Here's how the part is built. I have some questions about the finished solid (model axes, mm). Face numbers are marked on the shaded views. A direction names the side the tool comes from. Give positions to 0.01 mm unless a question says otherwise; leave off trailing zeros. Order: outer loops, then holes, each group sorted by start corner. A loop starts at its lowest first (then second) coordinate and runs counter-clockwise, first axis right, second up.
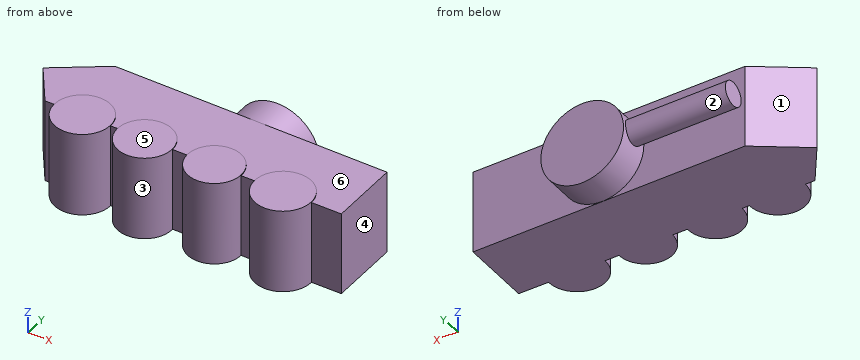
from build123d import *

# Parameters (mm, degrees)
F1_DEPTH = 39.081264
F2_R     = 13.086834
F2_R_2   = 12.762308
F2_R_3   = 12.541297
F2_R_4   = 13.219685
F3_DEPTH = 39.425768
F4_R     = 19.429487
F5_DEPTH = 14.579227
F6_R     = 5.692601
F7_DEPTH = 52.206531


with BuildPart() as f1:
    # F0 (on Top) → F1 (new body)
    with BuildSketch(Plane.XY):
        Polygon((-52.925434, 16.347141), (-76.083884, 0), (-63.54259, -17.766833), (74.829757, -16.512707), (74.829757, 16.347141), align=None)
    extrude(amount=F1_DEPTH)

    # F2 (on Top) → F3 (join)
    with BuildSketch(Plane.XY):
        with Locations((-45.984775, -17.766833)):
            Circle(F2_R)
        with Locations((-16.72174, -17.766833)):
            Circle(F2_R_2)
        with Locations((15.467599, -16.930744)):
            Circle(F2_R_3)
        with Locations((47.656953, -16.930744)):
            Circle(F2_R_4)
    extrude(amount=F3_DEPTH)

    # F4 (on face) → F5 (join)
    with BuildSketch(Plane(origin=(0, 16.347141, 0), x_dir=(-1, 0, 0), z_dir=(0, 1, 0))):
        with Locations((-14.022259, 19.540632)):
            Circle(F4_R)
    extrude(amount=F5_DEPTH)

    # F6 (on Right) → F7 (join)
    with BuildSketch(Plane.YZ):
        with Locations((23.680674, 21.317706)):
            Circle(F6_R)
    extrude(amount=-F7_DEPTH)


solid = f1.part
Q1. I'm going to push flat-ended pins straight in: P1, Ø10, axis at y = -8, z = 21.5, coming from the -X side; P2, Ø1.5, axis at y = 15.5, z = 16.5, coming from the -X side; P3, Ø8, axis at x = 5.5, z = 7.5, coming from the -Y side; P4, Ø10, axis at x = 5, y = -5, coming from the +Z side. Where does each tip first touch, or does it pass through?
Filled sheet:
P1: stops at x = -73.97
P2: stops at x = -55.19
P3: stops at y = -27.96
P4: stops at z = 39.43
Q2. For the marked faces 5 and 6, which set-ups out of +Z, -Z, +X, -X, +Y, -Y let a thin tool reach every point of the face, with its end or its side?
Filled sheet:
face 5: +Z, +X, -X, +Y, -Y
face 6: +Z, +Y
Q3. If we section it at B-B on x = -45: List the corners of the cut face in (y, z) for me, plus the area to 3 significant figures.
Filled sheet:
outline: (-30.82, 0) - (16.35, 0) - (16.35, 39.08) - (-4.72, 39.08) - (-4.72, 39.43) - (-30.82, 39.43) - close; circle Ø11.39 at (23.68, 21.32)
area: 1,950 mm2
Q4. If we section it at C-C on z = 32: List the corners of the cut face in (x, y) for me, plus the area to 3 significant figures.
Filled sheet:
outline: (-76.08, 0) - (-63.54, -17.77) - (-59.07, -17.73) arc R13.09 ccw (long way) to (-32.9, -17.49) - (-29.48, -17.46) arc R12.76 ccw (long way) to (-3.97, -17.23) - (2.93, -17.16) arc R12.54 ccw to (28.01, -16.94) - (34.44, -16.88) arc R13.22 ccw (long way) to (60.87, -16.64) - (74.83, -16.51) - (74.83, 16.35) - (28.93, 16.35) - (28.93, 30.93) - (-0.89, 30.93) - (-0.89, 16.35) - (-52.93, 16.35) - close
area: 6,260 mm2
Q5. Thinking about a two-plate mould opening in X: for the marked faces 1, 2, 3 and 4, which applies, released by +X, released by -X, zero draft, split by the parting line, or undercut?
Filled sheet:
face 1: released by -X
face 2: zero draft
face 3: undercut
face 4: released by +X
Q6. If we section it at D-D on x = -17: List the corners of the cut face in (y, z) for me, plus the area to 3 significant figures.
Filled sheet:
outline: (-30.53, 0) - (16.35, 0) - (16.35, 39.08) - (-5.01, 39.08) - (-5.01, 39.43) - (-30.53, 39.43) - close; circle Ø11.39 at (23.68, 21.32)
area: 1,940 mm2
Q7. I need wall thicknesses on L1, parallel to X at y = -24, z = 27.5; L2, parallel to Y at x = -15.5, z = 17.5; L3, parallel to X at y = -25, z = 35. Which ranges of each line are inside material? Lowest first, please.
Filled sheet:
L1: x = -57.49 to -34.48, -27.86 to -5.59, 5.11 to 25.83, 36.49 to 58.83
L2: y = -30.47 to 16.35, 19.46 to 27.9
L3: x = -56.89 to -35.08, -27.24 to -6.21, 5.87 to 25.07, 37.19 to 58.13
Q8. If we section it at A-A on y = -26.5: List the corners of the cut face in (x, z) for me, plus the area to 3 significant figures.
Filled sheet:
outline: (-55.73, 0) - (-36.24, 0) - (-36.24, 39.43) - (-55.73, 39.43) - close; (-26.03, 0) - (-7.42, 0) - (-7.42, 39.43) - (-26.03, 39.43) - close; (7.36, 0) - (23.57, 0) - (23.57, 39.43) - (7.36, 39.43) - close; (38.54, 0) - (56.78, 0) - (56.78, 39.43) - (38.54, 39.43) - close
area: 2,860 mm2
